Input: part model. Units: mm. Frame: model coordinates. A direction names the side the tool comes from. Coordinates: 2 decimals unless noted, no trailing zeros. Loops run counter-clockwise (first coordinate to the right, second up) from the corner with the lowest first, then second, coordinate; pieces in that order, holes last. Notation, with made-up numbers: (87, 70.5) - (135, 70.5) arc R22 cw to (135, 105.5) - close; hole circle Ø7 at (-10.75, -6). An arc over 180 degrees is marked (long way). Answer as CSV lines item,"result". Start each with the question number.
```python
from build123d import *

# Parameters (mm, degrees)
F1_DEPTH = 1160


with BuildPart() as f1:
    # F0 (on Front) → F1 (new body)
    with BuildSketch(Plane.XZ):
        with BuildLine():
            ThreePointArc((50, 45), (48.535534, 48.535534), (45, 50))
            Line((45, 50), (-45, 50))
            ThreePointArc((-45, 50), (-48.535534, 48.535534), (-50, 45))
            Line((-50, 45), (-50, -45))
            ThreePointArc((-50, -45), (-48.535534, -48.535534), (-45, -50))
            Line((-45, -50), (45, -50))
            ThreePointArc((45, -50), (48.535534, -48.535534), (50, -45))
            Line((50, -45), (50, 45))
        make_face()
        with BuildLine():
            ThreePointArc((-47, 45), (-46.414214, 46.414214), (-45, 47))
            Line((-45, 47), (45, 47))
            ThreePointArc((45, 47), (46.414214, 46.414214), (47, 45))
            Line((47, 45), (47, -45))
            ThreePointArc((47, -45), (46.414214, -46.414214), (45, -47))
            Line((45, -47), (-45, -47))
            ThreePointArc((-45, -47), (-46.414214, -46.414214), (-47, -45))
            Line((-47, -45), (-47, 45))
        make_face(mode=Mode.SUBTRACT)
    extrude(amount=-F1_DEPTH)


solid = f1.part
```
Item 1: Set-up query: faces 1 (the flat face through (-50, 572, 1)), 2 (the flat face through (-47, 572, -1)). Return all of +Z, -Z, +X, -X, +Y, -Y with unobstructed straight access to the full face (end or side cutting, diameter ignored); none if empty.
Item 2: Section query C-C, the plane y = 1040.5. Output: boundary loops of the cut face in (x, z).
Item 3: Section query A-A, the plane x = 7.5. Output: boundary loops of the cut face in (y, z), and give its area (3 significant figures).
Item 4: Section query B-B, the plane z = 24. Output: boundary loops of the cut face in (x, y), and give its area (3 significant figures).
Item 5: Draft query along X for faces 3 (the flat face through (50, 572, -1)), 4 (the flat face through (-1, 572, 47)), 5 (the flat face through (-1, 572, -50)). Return one class per face: pulls with the +X half, pulls with the -X half, needs draft (parallel to the pull), parting line crosses it, or undercut.
Item 6: Material intervals for probe 1 along Z at (x, y) = (-45, 667), sorted ascending.
Response values:
1,face 1,"+Z, -Z, -X, +Y, -Y"
1,face 2,"+Y, -Y"
2,outline,"(-50, -45) arc R5 ccw to (-45, -50) - (45, -50) arc R5 ccw to (50, -45) - (50, 45) arc R5 ccw to (45, 50) - (-45, 50) arc R5 ccw to (-50, 45) - close; hole (-47, -45) arc R2 ccw to (-45, -47) - (45, -47) arc R2 ccw to (47, -45) - (47, 45) arc R2 ccw to (45, 47) - (-45, 47) arc R2 ccw to (-47, 45) - close"
3,outline,"(0, -50) - (1160, -50) - (1160, -47) - (0, -47) - close; (0, 47) - (1160, 47) - (1160, 50) - (0, 50) - close"
3,area,"6,960 mm²"
4,outline,"(-50, 0) - (-47, 0) - (-47, 1160) - (-50, 1160) - close; (47, 0) - (50, 0) - (50, 1160) - (47, 1160) - close"
4,area,"6,960 mm²"
5,face 3,"pulls with the +X half"
5,face 4,"undercut"
5,face 5,"needs draft"
6,probe 1,"z = -50 to -47, 47 to 50"
